For this review, take the finished solid that the model builds, in its own axes (mm). Face numbers are marked on the shaded views. A direction names the side the tool comes from. Round coordinates to 2 decimals unless told otherwise and drop trailing zeros. Write each loop counter-clockwise with the first axis right and the second up, starting at its lowest first coordinate (ties: lowest second). Pieces come first, ordered by that corner, then holes. Notation, with made-up numbers: M 46,18 L 52,18 A21 cw 52,25 Z; hole C 5,-27.5 d6. An arc over 180 degrees is marked long. Use one line per item in the form item = value. Start each with the question number.
Item 1: Draft analysis for pull direction Y (two halves, no side actions). For the marked faces 1, 2 and 3, state which applies: released by +Y, released by -Y, zero draft, split by the parting line, or undercut.
Item 2: Add section B-B (z = 1.25). State the section outline as (x, y) points (3 decimals).
Item 3: Add section D-D (z = 4.75). State the section outline as (x, y) points (3 decimals), and give its area (3 significant figures).
Item 4: For P1, Ø19, axis at x = -4.5, y = 2.5, coming from the +Z side; P2, Ø1, axis at y = -4, z = 1, coming from the -X side; P3, Ø1, axis at y = 18, z = 2, coming from the -X side; P4, Ø12, axis at x = -6.5, y = 22.5, coming from the +Z side, all flat-tipped, find the tip position at first contact; note any pin that passes through.
Item 5: For line 1 (Y direction, x = 16.5, z = 2.5); line 2 (Z direction, x = -2, y = 0.5) (3 decimals); line 3 (X direction, y = -6.5, z = -1.75), list the stretches that pass through material, from the lowest coordinate up. Write a range as [from, to].
Item 6: For the marked faces 4 and 5, list the 3-axis set-ups (+Z, -Z, +X, -X, +Y, -Y) from which the entire face can be reached by the end or side of a thin tool; tool diameter is ignored.
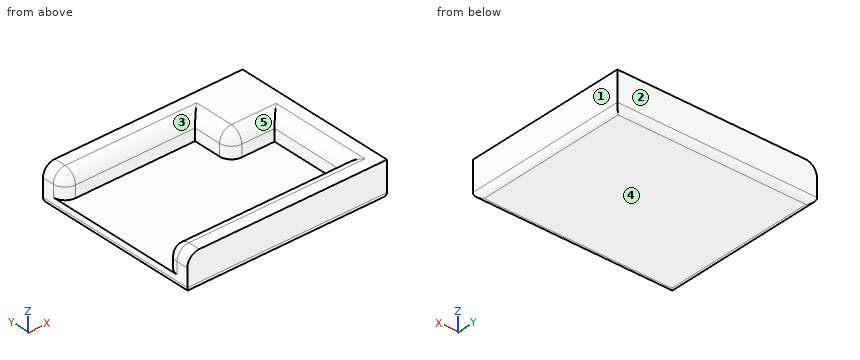
from build123d import *

# Parameters (mm, degrees)
F1_DEPTH = 3.175
F2_DEPTH = 6.35
F3_R     = 3.175
F4_R     = 3.175
F5_R     = 1.5875


with BuildPart() as f1:
    # F0 (on Top) → F1 (new body)
    with BuildSketch(Plane.XY):
        Polygon((8.5, 10.5), (20.5, 10.5), (20.5, -10.5), (-20.5, -10.5), (-26.85, -10.5), (-26.85, -16.85), (26.85, -16.85), (26.85, 27.6), (-26.85, 27.6), (-26.85, 21.25), (-20.5, 21.25), (8.5, 21.25), align=None)
        Polygon((20.5, -10.5), (20.5, 10.5), (8.5, 10.5), (8.5, 21.25), (-20.5, 21.25), (-20.5, 10.5), (-20.5, -10.5), align=None)
        Polygon((-26.85, -10.5), (-20.5, -10.5), (-20.5, 10.5), (-20.5, 21.25), (-26.85, 21.25), align=None)
    extrude(amount=-F1_DEPTH)

    # F0 (on Top) → F2 (join)
    with BuildSketch(Plane.XY):
        Polygon((8.5, 10.5), (20.5, 10.5), (20.5, -10.5), (-20.5, -10.5), (-26.85, -10.5), (-26.85, -16.85), (26.85, -16.85), (26.85, 27.6), (-26.85, 27.6), (-26.85, 21.25), (-20.5, 21.25), (8.5, 21.25), align=None)
    extrude(amount=F2_DEPTH)

    # F3
    f3_edges = [f1.edges().sort_by_distance(p)[0] for p in [
        (8.5, 10.5, 3.175),
        (-26.85, -10.5, 3.175),
        (-26.85, 21.25, 3.175),
    ]]
    fillet(f3_edges, radius=F3_R)

    # F4
    f4_edges = [f1.edges().sort_by_distance(p)[0] for p in [
        (9.429936, 11.429936, 6.35),
        (20.5, 0, 6.35),
        (-1.5875, -10.5, 6.35),
        (-7.5875, 21.25, 6.35),
    ]]
    fillet(f4_edges, radius=F4_R)

    # F5
    f5_edges = [f1.edges().sort_by_distance(p)[0] for p in [
        (0, -16.85, -3.175),
        (26.85, 5.375, -3.175),
        (0, 27.6, -3.175),
        (-26.85, 5.375, -3.175),
    ]]
    fillet(f5_edges, radius=F5_R)


solid = f1.part
Calculated:
q1.face_1 = zero draft
q1.face_2 = released by +Y
q1.face_3 = undercut
q2.outline = M -26.85,-16.85 L 26.85,-16.85 L 26.85,27.6 L -26.85,27.6 L -26.85,24.425 A3.175 ccw -23.675,21.25 L 8.5,21.25 L 8.5,13.675 A3.175 ccw 11.675,10.5 L 20.5,10.5 L 20.5,-10.5 L -23.675,-10.5 A3.175 ccw -26.85,-13.675 Z
q3.outline = M -26.432,-16.85 L 26.85,-16.85 L 26.85,27.6 L -26.432,27.6 L -26.432,24.425 A2.757 ccw -23.675,21.668 L 8.918,21.668 L 8.918,13.675 A2.757 ccw 11.675,10.918 L 20.918,10.918 L 20.918,-10.918 L -23.675,-10.918 A2.757 ccw -26.432,-13.675 Z
q3.area = 950 mm^2
q4.P1 = 0
q4.P2 = 20.5
q4.P3 = 8.5
q4.P4 = 6.35
q5.line_1 = [-16.85, -10.5], [10.5, 27.6]
q5.line_2 = [-3.175, 0]
q5.line_3 = [-26.84, 26.84]
q6.face_4 = -Z, +X, -X, +Y, -Y
q6.face_5 = +Z, -X
